from build123d import *

# Parameters (mm, degrees)
F1_DEPTH = 3
F3_DEPTH = 5
F4_R     = 3.95
F5_DEPTH = 3.5
F6_R     = 2.1
F7_DEPTH = 25
F8_R     = 5.510522
F8_R_2   = 3.95
F9_DEPTH = 0.5


with BuildPart() as f1:
    # F0 (on Top) → F1 (new body)
    with BuildSketch(Plane.XY):
        with BuildLine():
            ThreePointArc((-50, 10.487979), (-61.5, -1.012021), (-50, -12.512021))
            Line((-50, -12.512021), (0, -12.512021))
            Line((0, -12.512021), (50, -12.512021))
            ThreePointArc((50, -12.512021), (61.5, -1.012021), (50, 10.487979))
            ThreePointArc((50, 10.487979), (46.593573, 9.971888), (43.49289, 8.469937))
            ThreePointArc((43.49289, 8.469937), (40.537466, 7.038348), (37.290622, 6.546434))
            Line((37.290622, 6.546434), (0, 6.546434))
            Line((0, 6.546434), (-37.290622, 6.546434))
            ThreePointArc((-37.290622, 6.546434), (-40.537466, 7.038348), (-43.49289, 8.469937))
            ThreePointArc((-43.49289, 8.469937), (-46.593573, 9.971888), (-50, 10.487979))
        make_face()
    extrude(amount=F1_DEPTH)

    # F2 (on face) → F3 (join)
    with BuildSketch(Plane.XY):
        with BuildLine():
            ThreePointArc((-63.5, -1.012021), (-59.545942, -10.557963), (-50, -14.512021))
            Line((-50, -14.512021), (50, -14.512021))
            ThreePointArc((50, -14.512021), (59.545942, -10.557963), (63.5, -1.012021))
            Line((63.5, -1.012021), (61.5, -1.012021))
            ThreePointArc((61.5, -1.012021), (58.131728, -9.143749), (50, -12.512021))
            Line((50, -12.512021), (-50, -12.512021))
            ThreePointArc((-50, -12.512021), (-58.131728, -9.143749), (-61.5, -1.012021))
            Line((-61.5, -1.012021), (-63.5, -1.012021))
        make_face()
    extrude(amount=F3_DEPTH)

    # F4 (on face) → F5 (join)
    with BuildSketch(Plane.XY.offset(3)):
        with Locations((-50, -1.012021)):
            Circle(F4_R)
        with Locations((50, -1.012021)):
            Circle(F4_R)
    extrude(amount=F5_DEPTH)

    # F6 (on face) → F7 (cut)
    with BuildSketch(Plane.XY.offset(6.5)):
        with Locations((-50, -1.012021)):
            Circle(F6_R)
        with Locations((50, -1.012021)):
            Circle(F6_R)
    extrude(amount=-F7_DEPTH, mode=Mode.SUBTRACT)

    # F8 (on face) → F9 (join)
    with BuildSketch(Plane.XY.offset(3)):
        with Locations((-50, -1.012021)):
            Circle(F8_R)
        with Locations((-50, -1.012021)):
            Circle(F8_R_2, mode=Mode.SUBTRACT)
        with Locations((50, -1.012021)):
            Circle(F8_R)
        with Locations((50, -1.012021)):
            Circle(F8_R_2, mode=Mode.SUBTRACT)
    extrude(amount=F9_DEPTH)


solid = f1.part
Verification items for the finished model (mm, model axes). A direction names the side the tool comes from. Give positions to 0.01 mm unless a question says otherwise; leave off trailing zeros. Write each loop counter-clockwise with the first axis right and the second up, starting at its lowest first coordinate (ties: lowest second). Pieces come first, ordered by that corner, then holes. Notation, with made-up numbers: M 52,27 L 103,27 A14 ccw 103,33 Z; hole C -10,89.5 d7. An arc over 180 degrees is marked long. Use CSV: the item, a comma, the result in double quotes.
1) Access from +Z, -Z, +X, -X, +Y, -Y to the whole of each face (thin tool, end or side, straight path). Record for faces 1 (the face through (-1, -2, 0)), 2 (the face through (-48, -3, 6.5)), 3 (the face through (46, 0, 3.5)), 4 (the face through (-62, -1.012, 2)), 5 (the face through (-40.493, 7.025, 1.479)).
Final values:
face 1,"-Z, +X, -X, +Y, -Y"
face 2,"+Z, +X, -X, +Y, -Y"
face 3,"+Z"
face 4,"+Z, -Z, -X, +Y"
face 5,"+Z, -Z, +Y"
2) Cross-section at A-A (y = -9). Enter the section's corners in (x, z).
Final values:
outline,"M -60.88,0 L 60.88,0 L 60.88,5 L 58.27,5 L 58.27,3 L -58.27,3 L -58.27,5 L -60.88,5 Z"
3) Release check for a two-part mould opening along Y. For faces 6 (the face through (58.221, -9.054, 3.986)), 7 (the face through (52, -3, 6.5)), 8 (the face through (-1, -14.512, 2)), 9 (the face through (63, -1.012, 2)) record: released by +Y, released by -Y, zero draft, split by the parting line, or undercut.
Final values:
face 6,"undercut"
face 7,"zero draft"
face 8,"released by -Y"
face 9,"released by +Y"
4) Material ranges on line 1 along X through (y, z) = (-0.5, 1.75); line 2 along Y through (x, z) = (50, 2.25); line 3 along Y through (x, z) = (15, 0.75), recorded low to high.
Final values:
line 1,"-61.49 to -52.04, -47.96 to 47.96, 52.04 to 61.49"
line 2,"-14.51 to -3.11, 1.09 to 10.49"
line 3,"-14.51 to 6.55"
5) Go/stop test with flat-tipped pins: pin 1 Ø0.6 at (x, z) = (62.5, 2.5) entering from +Y; pin 2 Ø0.9 at (x, z) = (4, 1.5) entering from +Y; pin 3 Ø11 at (x, y) = (-29.5, -9) entering from +Z; pin 4 Ø4 at (x, y) = (-50, -1.01) entering from +Z. Record where each tip stops, or that it passes through.
Final values:
pin 1,"y = -1.01"
pin 2,"y = 6.55"
pin 3,"z = 5"
pin 4,"through"
6) Cross-section at B-B (x = -6.5). Enter the section's corners in (y, z), plus the area to 3 significant figures.
Final values:
outline,"M -14.51,0 L 6.55,0 L 6.55,3 L -12.51,3 L -12.51,5 L -14.51,5 Z"
area,"67.2 mm²"
